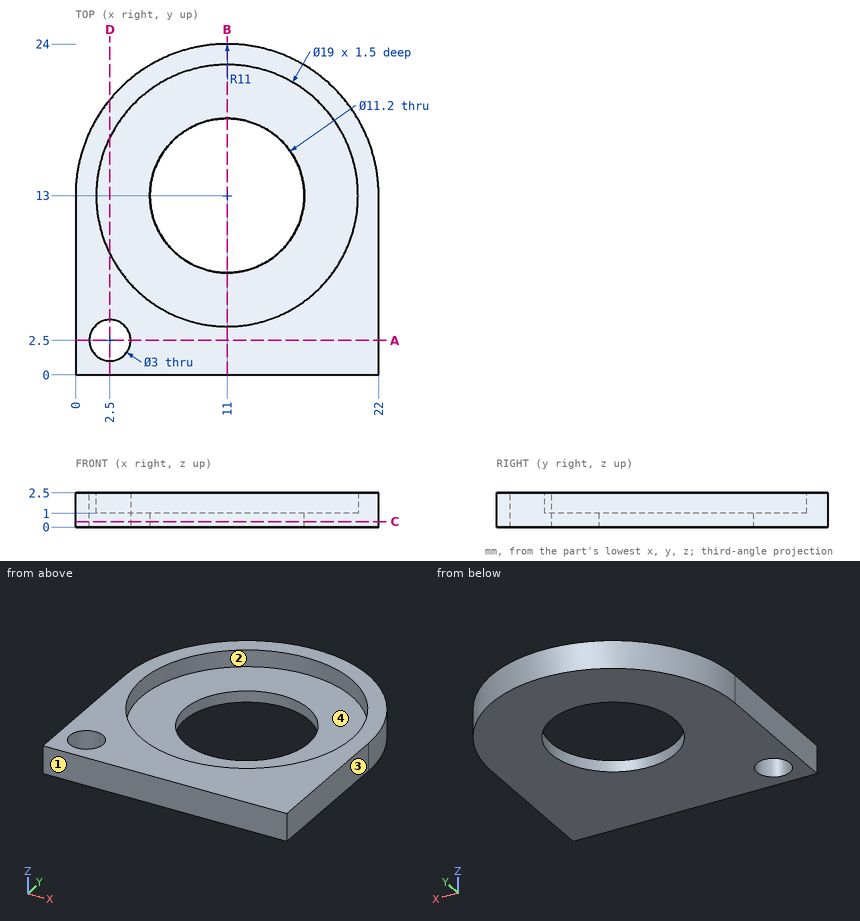
Could you check a few things on this drawing? It's one solid part, dimensions in mm from its lowest x, y, z. Round coordinates to 2 decimals unless told otherwise and drop trailing zeros. Loops run counter-clockwise (first coordinate to the right, second up) from the corner with the lowest first, then second, coordinate; pieces in that order, holes last. Notation, with made-up numbers: M -11.75,34.5 L 42.25,34.5 A11 cw 42.25,55.5 Z; hole C 3,-25 d11. An arc over 180 degrees is marked long. Write item = value, one per line. Start each with the question number.
(1) I need wall thicknesses on line 1 along X through (y, z) = (13, 0.75); line 2 along Y through (x, z) = (2.5, 1.7); line 3 along Y through (x, z) = (11.25, 2.2). Which ranges of each line are inside material? Lowest first, please.
(2) I'm going to push flat-ended pins straight in: P1, Ø10, axis at x = 8, y = 12, coming from the -Z side; P2, Ø3, axis at x = 7, y = 15, coming from the +Z side; P3, Ø2.5, axis at x = 2.5, y = 2.5, coming from the +Z side. Where does each tip first touch, or does it pass through?
(3) Suppose I cut it at A-A on y = 2.5. Write out the boundary of the cut face in (x, z), plus the area to 3 significant figures.
(4) If we mould it in two halves opening along X, with no side actions, what happens to the marked faces 1, 2, 3 and 4? For each: released by +X, released by -X, zero draft, split by the parting line, or undercut.
(5) Suppose I cut it at C-C on z = 0.4. Write out the boundary of the cut face in (x, y), plus the area to 3 significant figures.
(6) Suppose I cut it at B-B on x = 11. Write out the boundary of the cut face in (y, z).
(7) Suppose I cut it at D-D on x = 2.5. Write out the boundary of the cut face in (y, z), plus the area to 3 significant figures.
Answer block:
q1.line_1 = 0 to 5.4, 16.6 to 22
q1.line_2 = 0 to 1, 4 to 8.76, 17.24 to 19.98
q1.line_3 = 0 to 3.5, 22.5 to 24
q2.P1 = 0
q2.P2 = 1
q2.P3 = through
q3.outline = M 0,0 L 1,0 L 1,2.5 L 0,2.5 Z; M 4,0 L 22,0 L 22,2.5 L 4,2.5 Z
q3.area = 47.5 mm²
q4.face_1 = zero draft
q4.face_2 = undercut
q4.face_3 = released by +X
q4.face_4 = undercut
q5.outline = M 0,0 L 22,0 L 22,13 A11 ccw 0,13 Z; hole C 2.5,2.5 d3; hole C 11,13 d11.2
q5.area = 370 mm²
q6.outline = M 0,0 L 7.4,0 L 7.4,1 L 3.5,1 L 3.5,2.5 L 0,2.5 Z; M 18.6,0 L 24,0 L 24,2.5 L 22.5,2.5 L 22.5,1 L 18.6,1 Z
q7.outline = M 0,0 L 1,0 L 1,2.5 L 0,2.5 Z; M 4,0 L 19.98,0 L 19.98,2.5 L 17.24,2.5 L 17.24,1 L 8.76,1 L 8.76,2.5 L 4,2.5 Z
q7.area = 29.7 mm²
